Verification items for the finished model (mm, model axes). Face numbers are marked on the shaded views. A direction names the side the tool comes from. Give positions to 0.01 mm unless a question says otherwise; leave off trailing zeros. Loops run counter-clockwise (first coordinate to the right, second up) from the corner with the lowest first, then second, coordinate; pieces in that order, holes last. Notation, with made-up numbers: (12, 4) - (42, 4) arc R28 cw to (42, 30) - close; hole circle Ø9 at (81.5, 65.25). An arc over 180 degrees is marked (long way). One line per item, written item: value. Start each with the question number.
1. Sectioned sample at B-B (x = 0). Record the cut outline in (y, z), plus the area to 3 significant figures.
2. Scan lines: L1, parallel to Z at x = 2.25, y = -10; L2, parallel to Z at x = 1.25, y = -6; L3, parallel to X at y = -9.75, z = -1. Record each from-to range of solid material in increasing order. Write a range as [from, to].
3. Sectioned sample at A-A (z = 0). Record the cut outline in (x, y).
4. Gauge pin test, flat ends, axial feed: pin 1 (1.5 mm diameter, centred on x = 9.5, z = 3.5, fed in from -Y); pin 2 (1 mm diameter, centred on x = 1.5, y = 8, fed in from -Z); pin 3 (1 mm diameter, centred on x = -6, z = -3, fed in from +Y). Record the tip position at first contact, or that the pin passes through.
5. Sectioned sample at D-D (z = -7.5). Record the cut outline in (x, y), plus the area to 3 significant figures.
6. Sectioned sample at C-C (y = 10). Record the cut outline in (x, z), plus the area to 3 significant figures.
7. Access from +Z, -Z, +X, -X, +Y, -Y to the whole of each face (thin tool, end or side, straight path). Record for the marked faces 1 and 2.
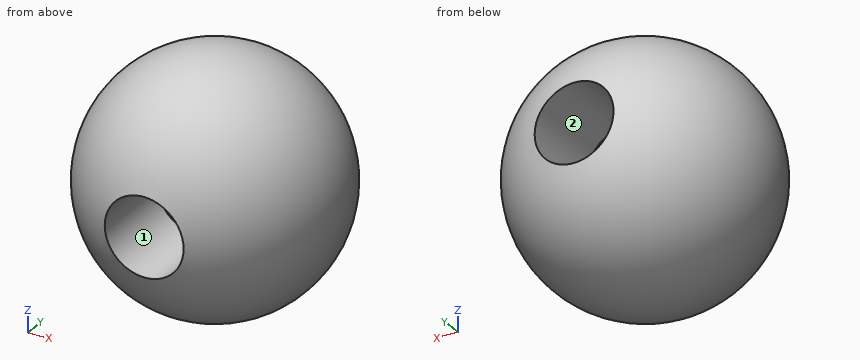
from build123d import *

# Parameters (mm, degrees)
SKIZZE3_R                       = 4
SCHNITT_LINEAR_AUSTRAGEN1_DEPTH = 20


with BuildPart() as part:
    # Skizze1 → Rotation1 (revolve)
    with BuildSketch(Plane.XY):
        with BuildLine():
            Line((0, 12.5), (0, -12.5))
            ThreePointArc((0, -12.5), (-12.5, 0), (0, 12.5))
        make_face()
    revolve(axis=Axis((0, 27.42628623, 0), (0, -1, 0)))

    # Skizze3 → Schnitt-Linear austragen1 (cut, symmetric)
    with BuildSketch(Plane(origin=(0, 0, 0), x_dir=(1, 0, 0), z_dir=(0, 1, 0))):
        Circle(SKIZZE3_R)
    extrude(amount=SCHNITT_LINEAR_AUSTRAGEN1_DEPTH, both=True, mode=Mode.SUBTRACT)

    # Skizze5 → Rotation2 (revolve)
    with BuildSketch(Plane(origin=(0, 0, 0), x_dir=(0, 0, -1), z_dir=(1, 0, 0))):
        Polygon((-2.15, 0), (-2.15, 2), (-5, 3.712452764), (-5, 0), align=None)
    rotation2 = revolve(axis=Axis((0, 0, 0), (0, 1, 0)))

    # Spiegeln1: Rotation2 across plane
    add(rotation2.mirror(Plane.ZX))


solid = part.part
Results are:
1. outline: (-11.84, -4) arc R12.5 ccw to (11.84, -4) - (3.11, -4) - (2, -2.15) - (-2, -2.15) - (-3.11, -4) - close; (-11.84, 4) - (-3.11, 4) - (-2, 2.15) - (2, 2.15) - (3.11, 4) - (11.84, 4) arc R12.5 ccw to start
1. area: 313 mm^2
2. L1: z = [-7.15, -3.31], [3.31, 7.15]
2. L2: z = [-10.89, -3.8], [3.8, 10.89]
2. L3: x = [-7.76, -3.87], [3.87, 7.76]
3. outline: (-4, -11.84) - (-4, -3.11) - (-2.15, -2) - (-2.15, 2) - (-4, 3.11) - (-4, 11.84) arc R12.5 ccw to start; (2.15, -2) - (4, -3.11) - (4, -11.84) arc R12.5 ccw to (4, 11.84) - (4, 3.11) - (2.15, 2) - close
4. pin 1: stops at y = -8.27
4. pin 2: stops at z = -9.89
4. pin 3: stops at y = 10.85
5. outline: circle Ø20 at (0, 0)
5. area: 314 mm^2
6. outline: circle Ø15 at (0, 0); hole circle Ø8 at (0, 0)
6. area: 126 mm^2
7. face 1: -Y
7. face 2: +Y
